from build123d import *

# Parameters (mm, degrees)
CHAMFER_1_SIZE = 0.5


with BuildPart() as part:
    # Эскиз1 → Повернуть1 (revolve)
    with BuildSketch(Plane.XY):
        Polygon((-98.05, 23), (-101.05, 23), (-101.05, 26), (-116.05, 26), (-116.05, 30), (-101.05, 30), (-101.05, 29), (-98.05, 29), align=None)
    revolve(axis=Axis((-108.55, 0, 0), (-1, 0, 0)))

    # Фаска1
    chamfer_1_edges = [part.edges().sort_by_distance(p)[0] for p in [
        (-116.05, -30, 0),
    ]]
    chamfer(chamfer_1_edges, length=CHAMFER_1_SIZE)


solid = part.part
Design review of the part built by this model. Coordinates are the model's own, in mm. A direction names the side the tool comes from. Round coordinates to 2 decimals unless told otherwise and drop trailing zeros. Write each loop counter-clockwise with the first axis right and the second up, starting at its lowest first coordinate (ties: lowest second). Pieces come first, ordered by that corner, then holes.
Item 1: For faces 1 (the flat face through (-116.05, -2, 26.1)), 2 (the flat face through (-101.05, -16, -25)), 3 (the cylindrical face through (-108.655, -20.633, 15.821)), list the 3-axis set-ups (+Z, -Z, +X, -X, +Y, -Y) from which the entire face can be reached by the end or side of a thin tool; tool diameter is ignored.
Item 2: Draft analysis for pull direction Y (two halves, no side actions). For faces 4 (the cylindrical face through (-99.53, 13.38, 25.73)), 5 (the flat face through (-98.05, -9, -22)), 6 (the flat face through (-101.05, -10, 21)), state which applies: released by +Y, released by -Y, zero draft, split by the parting line, or undercut.
Item 3: For pin 1 Ø5 at (x, z) = (-102.5, 5.5) entering from -Y; pin 2 Ø6 at (x, y) = (-114, -2) entering from -Z; pin 3 Ø5 at (x, y) = (-109.5, 6.5) entering from +Z; pin 4 Ø18 at (y, z) = (-3, 7) entering from +X, all flat-tipped, find the tip position at first contact; note any pin that passes through.
Item 4: Consider section A-A on z = 0. Give the boundary of the cut face in (x, y), and give its area (3 significant figures).
Item 5: Consider section C-C on x = -112. Give the boundary of the cut face in (y, z).
Item 6: Wall thickness on L1, parallel to Y at x = -100.05, z = 0; L2, parallel to Y at x = -112, z = 0: over which ranges is each line inside the solid? List them lowest first.
Check values:
1. face 1: +Z, -Z, -X, +Y, -Y
1. face 2: +X
1. face 3: -X
2. face 4: split by the parting line
2. face 5: zero draft
2. face 6: undercut
3. pin 1: stops at y = -29.85
3. pin 2: stops at z = -30
3. pin 3: stops at z = 29.73
3. pin 4: passes through
4. outline: (-116.05, -29.5) - (-115.55, -30) - (-101.05, -30) - (-101.05, -29) - (-98.05, -29) - (-98.05, -23) - (-101.05, -23) - (-101.05, -26) - (-116.05, -26) - close; (-116.05, 26) - (-101.05, 26) - (-101.05, 23) - (-98.05, 23) - (-98.05, 29) - (-101.05, 29) - (-101.05, 30) - (-115.55, 30) - (-116.05, 29.5) - close
4. area: 156 mm2
5. outline: circle Ø60 at (0, 0); hole circle Ø52 at (0, 0)
6. L1: y = -29 to -23, 23 to 29
6. L2: y = -30 to -26, 26 to 30
